Autodesk Inventor part; units mm, degrees
ref_plane "YZ Plane" through (0, 0, 0) normal (1, 0, 0) x (0, 1, 0)
ref_plane "XZ Plane" through (0, 0, 0) normal (0, 1, 0) x (-1, 0, 0)
ref_plane "XY Plane" through (0, 0, 0) normal (0, 0, 1) x (1, 0, 0)
sketch "Sketch1" plane through (0, 0, 0) normal (0, 1, 0) x (-1, 0, 0)
  line L0 (3, 0) -> (40.325, 0)
  line L1 (43.325, 3) -> (43.325, 13)
  line L2 (40.325, 16) -> (3, 16)
  line L3 (0, 13) -> (0, 3)
  circle A0 centre (17.525, 8) radius 6.625
  arc A1 (3, 16) -> (0, 13) centre (3, 13) ccw
  arc A2 (0, 3) -> (3, 0) centre (3, 3) ccw
  arc A3 (40.325, 0) -> (43.325, 3) centre (40.325, 3) ccw
  arc A4 (43.325, 13) -> (40.325, 16) centre (40.325, 13) ccw
  line L4 (10.9, 8) -> (17.525, 8)
  circle A5 centre (39.675, 8) radius 1.75
  point P0 (0, 0)
  point P1 (43.325, 16)
  point P2 (43.325, 0)
  point P3 (0, 16)
  dimension "d0" = 13.25
  dimension "d1" = 16
  dimension "d9" = 3
  dimension "d20" = 8
  dimension "d22" = 25.8
  dimension "d24" = 10.9
  dimension "d25" = 3.5
  dimension "d26" = 3.65
extrude "Extrusion1" add sketch "Sketch1" along normal blind 1.6
properties part number "PCBAux"
Can you work these out from the model? Positions are in its coordinate system, mm. Give positions to 0.01 mm unless a question says otherwise; leave off trailing zeros. Write each loop counter-clockwise with the first axis right and the second up, starting at its lowest first coordinate (ties: lowest second). Pieces come first, ordered by that corner, then holes. Notation, with made-up numbers: (25, -26) -> (73, -26) arc R22 cw to (73, -19) -> close; hole circle Ø1 at (52, 8.5). An arc over 180 degrees is marked (long way). One line per item, written item: value.
Q1. Imagine slicing it at B-B on x = -12. Please give me the cut outline in (y, z).
Results found:
outline: (0, 0) -> (1.6, 0) -> (1.6, 4.34) -> (0, 4.34) -> close; (0, 11.66) -> (1.6, 11.66) -> (1.6, 16) -> (0, 16) -> close
Q2. Please list where these lines run through material, in increasing order: line 1 (X direction, y = 1.15, z = 8.75) (3 decimals); line 2 (X direction, y = 1.15, z = 12.5) (3 decimals); line 3 (Z direction, x = -22, y = 0.2). Write a range as [from, to].
Results found:
line 1: x = [-43.325, -41.256], [-38.094, -24.107], [-10.943, 0]
line 2: x = [-43.325, -22.387], [-12.663, 0]
line 3: z = [0, 3.11], [12.89, 16]
Q3. Imagine slicing it at C-C on z = 14. Please give me the cut outline in (x, y).
Results found:
outline: (-43.15, 0) -> (-20.33, 0) -> (-20.33, 1.6) -> (-43.15, 1.6) -> close; (-14.72, 0) -> (-0.17, 0) -> (-0.17, 1.6) -> (-14.72, 1.6) -> close
Q4. For P1, Ø5, axis at x = -30, z = 12.5, coming from the -Y side, with a flat end and sliding along its axis, tell me the tip position at first contact or that it passes through.
Results found:
P1: stops at y = 0
Q5. Imagine slicing it at D-D on y = 0.5. Please give me the cut outline in (x, z) (3 decimals).
Results found:
outline: (-43.325, 3) arc R3 ccw to (-40.325, 0) -> (-3, 0) arc R3 ccw to (0, 3) -> (0, 13) arc R3 ccw to (-3, 16) -> (-40.325, 16) arc R3 ccw to (-43.325, 13) -> close; hole circle Ø3.5 at (-39.675, 8); hole circle Ø13.25 at (-17.525, 8)
Q6. We'd pull the mould along Z, two halves only. Please class faces 1 (the face through (0, 1, 8)), 2 (the face through (-22, 1, 16)), 3 (the face through (-41.29, 0.79, 8.67)): +Z half, -Z half, draft (parallel to the pull), parting line (faces both ways), or undercut.
Results found:
face 1: draft
face 2: +Z half
face 3: undercut
Q7. Imagine slicing it at A-A on z = 8. Please give me the cut outline in (x, y) (3 decimals).
Results found:
outline: (-43.325, 0) -> (-41.425, 0) -> (-41.425, 1.6) -> (-43.325, 1.6) -> close; (-37.925, 0) -> (-24.15, 0) -> (-24.15, 1.6) -> (-37.925, 1.6) -> close; (-10.9, 0) -> (0, 0) -> (0, 1.6) -> (-10.9, 1.6) -> close
